Could you check a few things on this drawing? It's one solid part, dimensions in mm from its lowest x, y, z. A direction names the side the tool comes from. Round coordinates to 2 decimals unless told otherwise and drop trailing zeros. Loops run counter-clockwise (first coordinate to the right, second up) from the corner with the lowest first, then second, coordinate; pieces in that order, holes last. Notation, with made-up numbers: M 52,43.25 L 95,43.25 A30 cw 95,66.25 Z; hole C -9.5,-23.75 d2. An arc over 180 degrees is marked long. Answer as a JSON object with one key per item and string values.
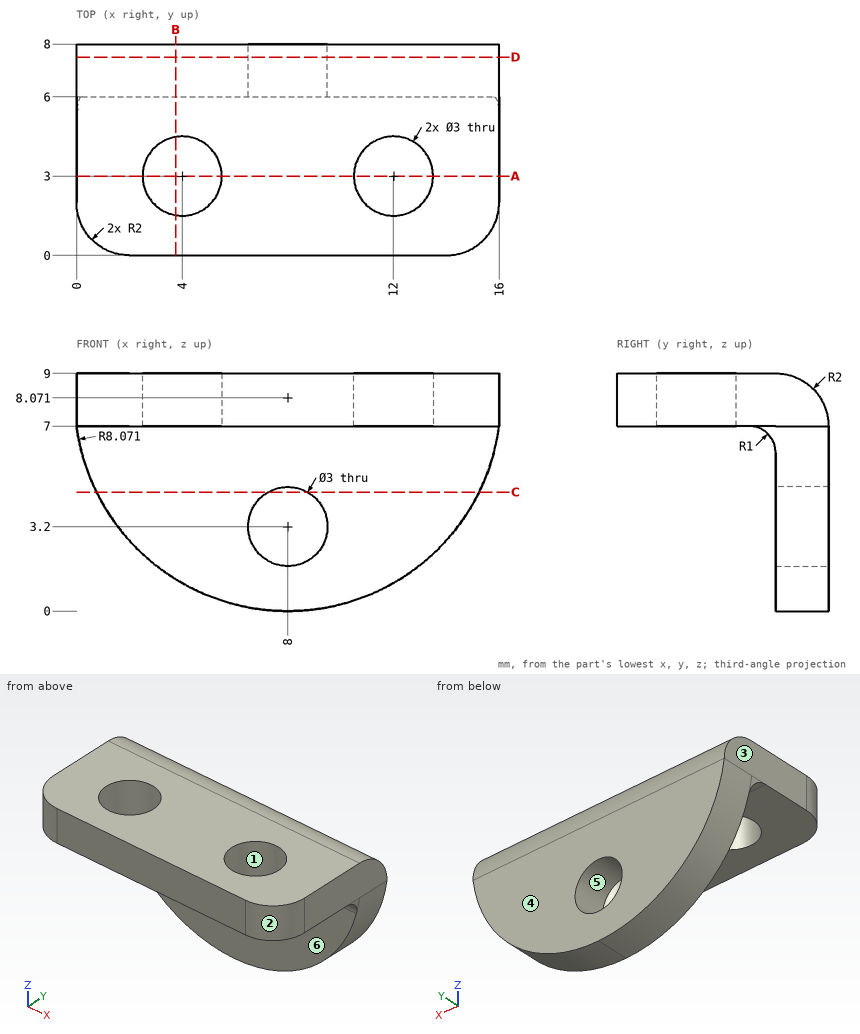
Item 1: If we mould it in two halves opening along Y, with no side actions, what happens to the marked faces 1, 2, 3 and 4? For each: pulls with the +Y half, pulls with the -Y half, needs draft (parallel to the pull), parting line crosses it, or undercut.
Resolved:
{"face 1": "undercut", "face 2": "pulls with the -Y half", "face 3": "needs draft", "face 4": "pulls with the +Y half"}
Item 2: I want a section at B-B, the plane x = 3.75. Please give me the cut outline in (y, z), then the cut area to 3 significant figures.
Resolved:
{"outline": "M 0,7 L 1.52,7 L 1.52,9 L 0,9 Z; M 4.48,7 L 5,7 A1 cw 6,6 L 6,1.21 L 8,1.21 L 8,7 A2 ccw 6,9 L 4.48,9 Z", "area": "21.0 mm²"}
Item 3: On a 3-axis mill with a long thin cutter (end or side, diameter ignored), from which of +Z, -Z, +X, -X, +Y, -Y can I reach the whole of each face in a straight line? I mean the marked faces 5 and 6. Say none if no direction works.
Resolved:
{"face 5": "+Y, -Y", "face 6": "-Z, +X, -X, -Y"}
Item 4: I want a section at D-D, the plane y = 7.5. Please give me the cut outline in (x, z).
Resolved:
{"outline": "M 0,7 A8.07 ccw 16,7 L 16,8.32 L 0,8.32 Z; hole C 8,3.2 d3"}
Item 5: Please list where these lines run through material, in increasing order: probe 1 along X at (y, z) = (2.25, 8.25); probe 2 along X at (y, z) = (3.5, 7.5) (1 decimal); probe 3 along Z at (x, y) = (9.5, 1). Write a range as from..to.
Resolved:
{"probe 1": "0..2.7, 5.3..10.7, 13.3..16", "probe 2": "0..2.6, 5.4..10.6, 13.4..16", "probe 3": "7..9"}
Item 6: I want a section at A-A, the plane y = 3. Please give me the cut outline in (x, z).
Resolved:
{"outline": "M 0,7 L 2.5,7 L 2.5,9 L 0,9 Z; M 5.5,7 L 10.5,7 L 10.5,9 L 5.5,9 Z; M 13.5,7 L 16,7 L 16,9 L 13.5,9 Z"}
Item 7: I want a section at C-C, the plane z = 4.5. Please give me the cut outline in (x, y).
Resolved:
{"outline": "M 0.76,6 L 7.25,6 L 7.25,8 L 0.76,8 Z; M 8.75,6 L 15.24,6 L 15.24,8 L 8.75,8 Z"}
Item 8: I'm going to push flat-ended pins straight in: pin 1 Ø3.5 at (x, y) = (4, 3) entering from -Z; pin 2 Ø3 at (x, z) = (4.5, 2.5) entering from -Y. Where does each tip first touch, or does it pass through?
Resolved:
{"pin 1": "z = 7", "pin 2": "y = 6"}
